Build history of the part. All positions in model axes, mm. Give positions to 0.01 mm unless a question says otherwise; leave off trailing zeros. Write each loop counter-clockwise with the first axis right and the second up, starting at its lowest first coordinate (ties: lowest second). Pieces come first, ordered by that corner, then holes. Notation, with made-up numbers: (67, -2) - (122, -2) arc R23 ccw to (122, 7) - close; hole circle Ø3 at (84, -8). An arc over 180 degrees is marked (long way). Use one line per item in the form item = value. Start each with the question number.
from build123d import *

# Parameters (mm, degrees)
F0_R     = 55
F0_R_2   = 52.5
F1_DEPTH = 500


with BuildPart() as f1:
    # F0 (on Front) → F1 (new body)
    with BuildSketch(Plane.XZ):
        Circle(F0_R)
        Circle(F0_R_2, mode=Mode.SUBTRACT)
    extrude(amount=F1_DEPTH)

    # F2 (on Right) → F3 (revolve, cut)
    with BuildSketch(Plane.YZ):
        Polygon((0, 49.5), (0, 55), (-5.5, 55), align=None)
    revolve(axis=Axis((0, 0, 0), (0, -1, 0)), mode=Mode.SUBTRACT)

    # F4 (on Right) → F5 (revolve, cut)
    with BuildSketch(Plane.YZ):
        Polygon((-500, 49.5), (-494.5, 55), (-500, 55), align=None)
    revolve(axis=Axis((0, -500, 0), (0, -1, 0)), mode=Mode.SUBTRACT)


solid = f1.part
(1) Two-plate mould, pull along X, no slides. Class faces 1 (the cylindrical face through (50.076, -246.542, 15.77)), 2 (the cylindrical face through (50.806, -246.577, -21.065)): +X half, -X half, draft (parallel to the pull), parting line (faces both ways), or undercut.
(2) Cut at A-A, the plane x = 0. Give the cut face in (y, z), then the cut area to 3 significant figures.
(3) Cut at C-C, the plane y = -238.5. Give the cut face in (x, z), then the cut area to 3 significant figures.
(4) Cut at B-B, the plane z = 0. Give the cut face in (x, y), then the cut area to 3 significant figures.
(5) Pin check, flat tips, straight feed: pin 1 Ø5 at (x, y) = (42, -407.5) entering from +Z; pin 2 Ø8 at (x, y) = (22, -423.5) entering from -Z; pin 3 Ø4 at (y, z) = (-137.5, -11.5) entering from -X. Stop position of each tip, or through.
(6) Wall check: line 1 (Z direction, x = 0, y = -338); line 2 (X direction, y = -370.5, z = -32.5). Give the ranges that are in metal, low to high. Write a range as from..to.
Solution:
q1.face_1 = undercut
q1.face_2 = parting line
q2.outline = (-497, -52.5) - (-494.5, -55) - (-5.5, -55) - (-3, -52.5) - close; (-497, 52.5) - (-3, 52.5) - (-5.5, 55) - (-494.5, 55) - close
q2.area = 2,460 mm2
q3.outline = circle Ø110 at (0, 0); hole circle Ø105 at (0, 0)
q3.area = 844 mm2
q4.outline = (-55, -494.5) - (-52.5, -497) - (-52.5, -3) - (-55, -5.5) - close; (52.5, -497) - (55, -494.5) - (55, -5.5) - (52.5, -3) - close
q4.area = 2,460 mm2
q5.pin_1 = 38.27
q5.pin_2 = -51.97
q5.pin_3 = -54.17
q6.line_1 = -55..-52.5, 52.5..55
q6.line_2 = -44.37..-41.23, 41.23..44.37
